```python
from build123d import *

# Parameters (mm, degrees)
BOSS_EXTRUDE1_DEPTH = 80
SKETCH2_W           = 7
SKETCH2_H           = 2
BOSS_EXTRUDE2_DEPTH = 5
BOSS_EXTRUDE3_DEPTH = 8
BOSS_EXTRUDE4_DEPTH = 8


with BuildPart() as part:
    # Sketch1 → Boss-Extrude1 (new body)
    with BuildSketch(Plane(origin=(0, 0, 0), x_dir=(1, 0, 0), z_dir=(0, 1, 0))):
        Polygon((-1.154700538, 2), (-2.309401077, 0), (-1.154700538, -2), (1.154700538, -2), (2.309401077, 0), (1.154700538, 2), align=None)
    extrude(amount=BOSS_EXTRUDE1_DEPTH)

    # Sketch2 → Boss-Extrude2 (add)
    with BuildSketch(Plane(origin=(0, 80, 0), x_dir=(1, 0, 0), z_dir=(0, 1, 0))):
        Rectangle(SKETCH2_W, SKETCH2_H)
    extrude(amount=-BOSS_EXTRUDE2_DEPTH)

    # Sketch3 → Boss-Extrude3 (add)
    with BuildSketch(Plane(origin=(0, 0, 0), x_dir=(0, 0, -1), z_dir=(1, 0, 0))):
        Polygon((-1.5, 6), (-0.5, 6), (1.5, 0), (0.5, 0), align=None)
    extrude(amount=BOSS_EXTRUDE3_DEPTH)

    # Sketch4 → Boss-Extrude4 (add)
    with BuildSketch(Plane(origin=(0, 0, 0), x_dir=(0, 0, -1), z_dir=(1, 0, 0))):
        Polygon((1.5, 6), (0.5, 6), (-1.5, 0), (-0.5, 0), align=None)
    extrude(amount=-BOSS_EXTRUDE4_DEPTH)


solid = part.part
```
Verification items for the finished model (mm, model axes). A direction names the side the tool comes from. Coordinates: 2 decimals unless noted, no trailing zeros. Loops run counter-clockwise (first coordinate to the right, second up) from the corner with the lowest first, then second, coordinate; pieces in that order, holes last. Notation, with made-up numbers: (-22.75, 32.5) -> (-0.75, 32.5) arc R15 ccw to (-0.75, 58.5) -> close; hole circle Ø5 at (33.5, 74.25). An arc over 180 degrees is marked (long way). Answer in a Markdown table with one row per item.
1) Depth check by flat-ended pin: P1, Ø4, axis at x = 4, y = 50.5, coming from the -Z side; P2, Ø1, axis at y = 77.5, z = 0, coming from the +X side; P3, Ø4, axis at x = 3.5, y = 44.5, coming from the -Z side. Enter the tip coordinate at first touch or a pass-through.
The answers:
| item | result |
|---|---|
| P1 | stops at z = -0.54 |
| P2 | stops at x = 3.5 |
| P3 | stops at z = -1.4 |
2) Scan lines: line 1 along X through (y, z) = (17, -1.8); line 2 along Z through (x, y) = (2.25, 56.5); line 3 along X through (y, z) = (51, 0.65). Record each from-to range of solid material in increasing order. Write a range as from..to.
The answers:
| item | result |
|---|---|
| line 1 | x = -1.27..1.27 |
| line 2 | z = -0.1..0.1 |
| line 3 | x = -1.93..1.93 |
3) Section check B-B (x = -5.75). Record the cut outline in (y, z).
The answers:
| item | result |
|---|---|
| outline | (0, 0.5) -> (6, -1.5) -> (6, -0.5) -> (0, 1.5) -> close |
4) Section check A-A (y = 49.5). Record the cut outline in (x, z), and give its area (3 significant figures).
The answers:
| item | result |
|---|---|
| outline | (-2.31, 0) -> (-1.15, -2) -> (1.15, -2) -> (2.31, 0) -> (1.15, 2) -> (-1.15, 2) -> close |
| area | 13.9 mm2 |
5) Draft check along Y on faces 5 (the face through (0, 0, 0)), 6 (the face through (1.724, 39.44, 1.014)), 7 (the face through (3.5, 78, 0)). Enter one of: released by +Y, released by -Y, zero draft, split by the parting line, or undercut.
The answers:
| item | result |
|---|---|
| face 5 | released by -Y |
| face 6 | undercut |
| face 7 | zero draft |
6) Access from +Z, -Z, +X, -X, +Y, -Y to the whole of each face (thin tool, end or side, straight path). Record for faces 1 (the face through (-3, 78, -1)), 2 (the face through (-3.5, 78, 0)), 3 (the face through (3, 78, -1)), 4 (the face through (3, 78, 1)).
The answers:
| item | result |
|---|---|
| face 1 | -Z, -X, +Y |
| face 2 | +Z, -Z, -X, +Y |
| face 3 | -Z, +X, +Y |
| face 4 | +Z, +X, +Y |
